Here's how the part is built. I have some questions about the finished solid (model axes, mm). Face numbers are marked on the shaded views. Give positions to 0.01 mm unless a question says otherwise; leave off trailing zeros. Order: outer loops, then holes, each group sorted by start corner. A loop starts at its lowest first (then second) coordinate and runs counter-clockwise, first axis right, second up.
from build123d import *

# Parameters (mm, degrees)
SKETCH1_R           = 44.45
BOSS_EXTRUDE1_DEPTH = 2.54
SKETCH2_R           = 38.1
SKETCH3_R           = 10.16
BOSS_EXTRUDE2_DEPTH = 3.175


with BuildPart() as part:
    # Sketch1 → Boss-Extrude1 (new body)
    with BuildSketch(Plane.XY):
        Circle(SKETCH1_R)
    extrude(amount=BOSS_EXTRUDE1_DEPTH)

    # Sketch2 → section 1 of loft1
    with BuildSketch(Plane.XY.offset(6.35), mode=Mode.PRIVATE) as loft1_s1:
        Circle(SKETCH2_R)
    # loft up to a face of the part (loft1)
    loft([Face(Wire([part.edges().sort_by_distance((-30.428118859, 32.402655489, 2.54))[0]])), loft1_s1.sketch])

    # Mirror3: part across plane


with BuildPart() as part_1:
    add(part.part)
    add(part.part.mirror(Plane.XY.offset(6.35)))

    # Sketch3 → Boss-Extrude2 (add)
    with BuildSketch(Plane.XY.offset(12.7)):
        with Locations(Location((0, 0, 0), (0, 0, 180))):
            Circle(SKETCH3_R)
    extrude(amount=BOSS_EXTRUDE2_DEPTH)


solid = part_1.part
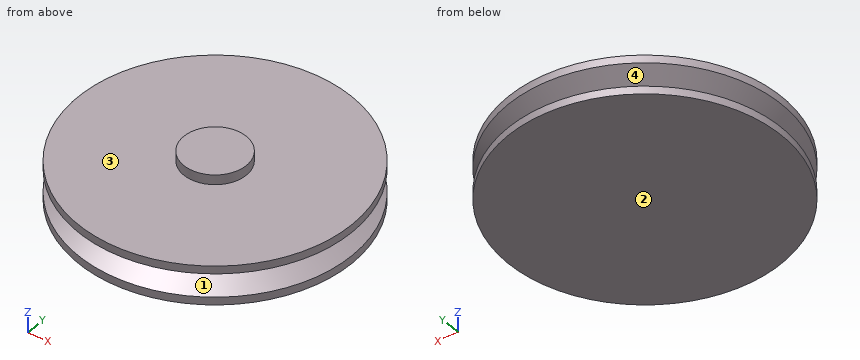
Q1. If we section it at B-B on z = 7.5: List the corners of the cut face in (x, y) for me.
Filled sheet:
outline: circle Ø80.03 at (0, 0)
Q2. I'm going to push flat-ended pins straight in: P1, Ø5, axis at x = -21.5, y = 29.5, coming from the -Z side; P2, Ø1.5, axis at x = 20.5, z = 8, coming from the -Y side; P3, Ø3, axis at x = 25, y = 2, coming from the +Z side; P4, Ø3, axis at y = 21, z = 3.5, coming from the -X side. Where does each tip first touch, or does it pass through?
Filled sheet:
P1: stops at z = 0
P2: stops at y = -36.83
P3: stops at z = 12.7
P4: stops at x = -39.77
Q3. I need wall thicknesses on L1, parallel to Z at x = -11.5, y = -34; L2, parallel to Y at x = -36, z = 11.5; L3, parallel to X at y = 29, z = 10.25. Which ranges of each line are inside material? Lowest first, please.
Filled sheet:
L1: z = 0 to 12.7
L2: y = -26.07 to 26.07
L3: x = -33.69 to 33.69
Q4. Thinking about a two-plate mould opening in Z: for the marked faces 1, 2, 3 and 4, which applies, released by +Z, released by -Z, zero draft, split by the parting line, or undercut?
Filled sheet:
face 1: undercut
face 2: released by -Z
face 3: released by +Z
face 4: undercut
Q5. If we section it at A-A on x = 0: List the corners of the cut face in (y, z) for me (3 decimals).
Filled sheet:
outline: (-44.45, 0) - (44.45, 0) - (44.45, 2.54) - (38.1, 6.35) - (44.45, 10.16) - (44.45, 12.7) - (10.16, 12.7) - (10.16, 15.875) - (-10.16, 15.875) - (-10.16, 12.7) - (-44.45, 12.7) - (-44.45, 10.16) - (-38.1, 6.35) - (-44.45, 2.54) - close
